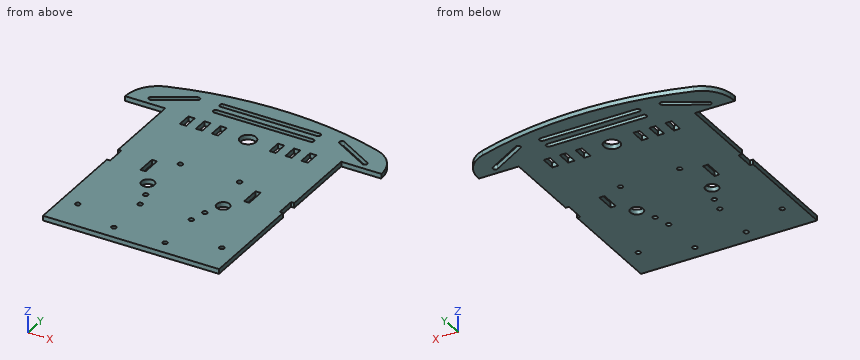
```python
from build123d import *

# Parameters (mm, degrees)
EXTRUDE_1_DEPTH     = 3
CUT_EXTRUDE_1_DEPTH = 133.037873355
SKETCH_3_W          = 2
SKETCH_3_H          = 12
SKETCH_3_W_2        = 3.2
CUT_EXTRUDE_2_DEPTH = 133.037873355
SKETCH_4_R          = 4
CUT_EXTRUDE_3_DEPTH = 133.037873355
SKETCH_5_R          = 5
SKETCH_5_W          = 4
SKETCH_5_H          = 9
CUT_EXTRUDE_4_DEPTH = 133.037873355
SKETCH_6_R          = 1.5
CUT_EXTRUDE_5_DEPTH = 10
SKETCH_8_R          = 1.5
CUT_EXTRUDE_7_DEPTH = 133.037873355
SKETCH_9_R          = 1.5
CUT_EXTRUDE_8_DEPTH = 133.037873355


with BuildPart() as part:
    # 草图1 → 凸台-拉伸1 (new body)
    with BuildSketch(Plane.XY):
        with BuildLine():
            Line((55, -55), (-55, -55))
            Line((-55, -55), (-55, 75))
            Line((-55, 75), (-80, 75))
            ThreePointArc((-80, 75), (-79.917609458, 77.027988882), (-79.670980888, 79.042610796))
            ThreePointArc((-79.670980888, 79.042610796), (-75.043492411, 88.912306625), (-65.927615795, 94.889374375))
            ThreePointArc((-65.927615795, 94.889374375), (0, 105), (65.927615795, 94.889374375))
            ThreePointArc((65.927615795, 94.889374375), (75.043492411, 88.912306625), (79.670980888, 79.042610796))
            ThreePointArc((79.670980888, 79.042610796), (79.917609458, 77.027988882), (80, 75))
            Line((80, 75), (55, 75))
            Line((55, 75), (55, -55))
        make_face()
    extrude(amount=EXTRUDE_1_DEPTH)

    # 草图2 → 切除-拉伸1 (cut, through all)
    with BuildSketch(Plane(origin=(0, 0, 0), x_dir=(-1, 0, 0), z_dir=(0, 0, -1))):
        with BuildLine():
            Line((-30, 94.5), (30, 94.5))
            ThreePointArc((30, 94.5), (31.5, 93), (30, 91.5))
            Line((30, 91.5), (-30, 91.5))
            ThreePointArc((-30, 91.5), (-31.5, 93), (-30, 94.5))
        make_face()
        with BuildLine():
            Line((-67.497284367, 81.299038106), (-45.846649273, 93.799038106))
            ThreePointArc((-45.846649273, 93.799038106), (-43.797611167, 93.25), (-44.346649273, 91.200961894))
            Line((-44.346649273, 91.200961894), (-65.997284367, 78.700961894))
            ThreePointArc((-65.997284367, 78.700961894), (-68.046322473, 79.25), (-67.497284367, 81.299038106))
        make_face()
        with BuildLine():
            Line((65.997284367, 78.700961894), (44.346649273, 91.200961894))
            ThreePointArc((44.346649273, 91.200961894), (43.797611167, 93.25), (45.846649273, 93.799038106))
            Line((45.846649273, 93.799038106), (67.497284367, 81.299038106))
            ThreePointArc((67.497284367, 81.299038106), (68.046322473, 79.25), (65.997284367, 78.700961894))
        make_face()
        with BuildLine():
            Line((-30, 87.5), (30, 87.5))
            ThreePointArc((30, 87.5), (31.5, 86), (30, 84.5))
            Line((30, 84.5), (-30, 84.5))
            ThreePointArc((-30, 84.5), (-31.5, 86), (-30, 87.5))
        make_face()
    extrude(amount=-CUT_EXTRUDE_1_DEPTH, mode=Mode.SUBTRACT)

    # 草图3 → 切除-拉伸2 (cut, through all)
    with BuildSketch(Plane.XY.offset(3)):
        with Locations((-54, 19)):
            Rectangle(SKETCH_3_W, SKETCH_3_H)
        with Locations((-32.4, 19)):
            Rectangle(SKETCH_3_W_2, SKETCH_3_H)
        with Locations((32.4, 19)):
            Rectangle(SKETCH_3_W_2, SKETCH_3_H)
        with Locations((54, 19)):
            Rectangle(SKETCH_3_W, SKETCH_3_H)
    extrude(amount=-CUT_EXTRUDE_2_DEPTH, mode=Mode.SUBTRACT)

    # 草图4 → 切除-拉伸3 (cut, through all)
    with BuildSketch(Plane(origin=(0, 0, 0), x_dir=(-1, 0, 0), z_dir=(0, 0, -1))):
        with Locations((23.5, 3)):
            Circle(SKETCH_4_R)
        with Locations(Location((-23.5, 3, 0), (0, 0, 180))):
            Circle(SKETCH_4_R)
    extrude(amount=-CUT_EXTRUDE_3_DEPTH, mode=Mode.SUBTRACT)

    # 草图5 → 切除-拉伸4 (cut, through all)
    with BuildSketch(Plane(origin=(0, 0, 0), x_dir=(-1, 0, 0), z_dir=(0, 0, -1))):
        with Locations((0, 69.5)):
            Circle(SKETCH_5_R)
        with Locations((-38, 69.5)):
            Rectangle(SKETCH_5_W, SKETCH_5_H)
        with Locations((-28, 69.5)):
            Rectangle(SKETCH_5_W, SKETCH_5_H)
        with Locations((-18, 69.5)):
            Rectangle(SKETCH_5_W, SKETCH_5_H)
        with Locations((18, 69.5)):
            Rectangle(SKETCH_5_W, SKETCH_5_H)
        with Locations((28, 69.5)):
            Rectangle(SKETCH_5_W, SKETCH_5_H)
        with Locations((38, 69.5)):
            Rectangle(SKETCH_5_W, SKETCH_5_H)
    extrude(amount=-CUT_EXTRUDE_4_DEPTH, mode=Mode.SUBTRACT)

    # 草图6 → 切除-拉伸5 (cut)
    with BuildSketch(Plane(origin=(0, 0, 0), x_dir=(-1, 0, 0), z_dir=(0, 0, -1))):
        with Locations((18.5, 29)):
            Circle(SKETCH_6_R)
        with Locations((18.5, -8)):
            Circle(SKETCH_6_R)
        with Locations((-18.5, -8)):
            Circle(SKETCH_6_R)
        with Locations((-18.5, 29)):
            Circle(SKETCH_6_R)
    extrude(amount=-CUT_EXTRUDE_5_DEPTH, mode=Mode.SUBTRACT)

    # 草图8 → 切除-拉伸7 (cut, through all)
    with BuildSketch(Plane(origin=(0, 0, 0), x_dir=(-1, 0, 0), z_dir=(0, 0, -1))):
        with Locations((-16, -46)):
            Circle(SKETCH_8_R)
        with Locations((-16, -18)):
            Circle(SKETCH_8_R)
        with Locations((16, -18)):
            Circle(SKETCH_8_R)
        with Locations((16, -46)):
            Circle(SKETCH_8_R)
    extrude(amount=-CUT_EXTRUDE_7_DEPTH, mode=Mode.SUBTRACT)

    # 草图9 → 切除-拉伸8 (cut, through all)
    with BuildSketch(Plane(origin=(0, 0, 0), x_dir=(-1, 0, 0), z_dir=(0, 0, -1))):
        with Locations((-45, -35)):
            Circle(SKETCH_9_R)
        with Locations((45, -35)):
            Circle(SKETCH_9_R)
    extrude(amount=-CUT_EXTRUDE_8_DEPTH, mode=Mode.SUBTRACT)


solid = part.part
```
Verification items for the finished model (mm, model axes). Give positions to 0.01 mm unless a question says otherwise; leave off trailing zeros. Write each loop counter-clockwise with the first axis right and the second up, starting at its lowest first coordinate (ties: lowest second). Pieces come first, ordered by that corner, then holes. Notation, with made-up numbers: M -21.75,75 L -16.75,75 A30 cw -16.75,105 Z; hole C 23.25,26.25 d5. An arc over 180 degrees is marked long. One line per question, with ' | ' between items.
1) Section check B-B on x = 10.5. Enter the section's corners in (y, z), plus the area to 3 significant figures.
Result:
outline: M -55,0 L 84.5,0 L 84.5,3 L -55,3 Z; M 87.5,0 L 91.5,0 L 91.5,3 L 87.5,3 Z; M 94.5,0 L 104.75,0 L 104.75,3 L 94.5,3 Z | area: 461 mm2
2) Gauge pin test, flat ends, axial feed: pin 1 Ø0.9 at (x, z) = (-19, 1.5) entering from +Y; pin 2 Ø0.9 at (x, z) = (-66, 1.5) entering from -Y; pin 3 Ø1.5 at (y, z) = (71, 1) entering from +X; pin 4 Ø5 at (x, y) = (23.5, 3) entering from +Z. Record the tip position at first contact, or that the pin passes through.
Result:
pin 1: stops at y = 104.22 | pin 2: stops at y = 75 | pin 3: stops at x = 55 | pin 4: passes through
3) Section check A-A on x = 60. Enter the section's corners in (y, z), plus the area to 3 significant figures.
Result:
outline: M 75,0 L 82.16,0 L 82.16,3 L 75,3 Z; M 85.63,0 L 96.66,0 L 96.66,3 L 85.63,3 Z | area: 54.6 mm2
4) Section check D-D on y = 1. Enter the section's corners in (x, z), plus the area to 3 significant figures.
Result:
outline: M -55,0 L -26.96,0 L -26.96,3 L -55,3 Z; M -20.04,0 L 20.04,0 L 20.04,3 L -20.04,3 Z; M 26.96,0 L 55,0 L 55,3 L 26.96,3 Z | area: 288 mm2
5) Section check C-C on z = 1.3. State how many separate pieces and enclosed holes the cut face has, plus the area to 3 significant figures.
Result:
separate pieces: 1 | enclosed holes: 25 | area: 17,100 mm2
6) Thickness scan on line 1 along Y through (x, z) = (0, 1.95); line 2 along X through (y, z) = (24.5, 1.95); line 3 along X through (y, z) = (-0.5, 2.45). Record the ranges inside material, lowest first. Write a range as [from, to].
Result:
line 1: y = [-55, 64.5], [74.5, 84.5], [87.5, 91.5], [94.5, 105] | line 2: x = [-53, -34], [-30.8, 30.8], [34, 53] | line 3: x = [-55, -25.44], [-21.56, 21.56], [25.44, 55]
